Verification items for the finished model (mm, model axes). Face numbers are marked on the shaded views. A direction names the side the tool comes from. Round coordinates to 2 decimals unless told otherwise and drop trailing zeros. Order: outer loops, then holes, each group sorted by start corner. A loop starts at its lowest first (then second) coordinate and runs counter-clockwise, first axis right, second up. Notation, with made-up numbers: M 8.5,60 L 55.5,60 A36 ccw 55.5,99 Z; hole C 46.5,20.5 d7. An arc over 180 degrees is marked long. One line per item, written item: value. Start each with the question number.
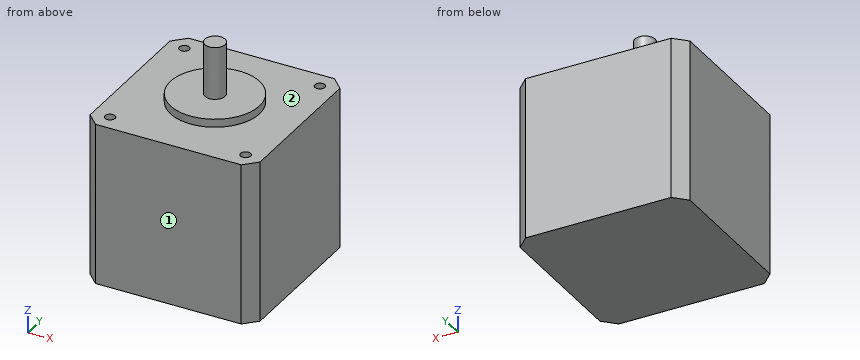
Autodesk Inventor part; units mm, degrees
ref_plane "YZ Plane" through (0, 0, 0) normal (1, 0, 0) x (0, 1, 0)
ref_plane "XZ Plane" through (0, 0, 0) normal (0, 1, 0) x (-1, 0, 0)
ref_plane "XY Plane" through (0, 0, 0) normal (0, 0, 1) x (1, 0, 0)
sketch "Sketch1" plane through (0, 0, 0) normal (0, 0, 1) x (1, 0, 0)
  line L0 (-3.9016, 5.1111) -> (32.0984, 5.1111)
  line L1 (35.0984, 2.1111) -> (35.0984, -33.8889)
  line L2 (32.0984, -36.8889) -> (-3.9016, -36.8889)
  line L3 (-6.9016, -33.8889) -> (-6.9016, 2.1111)
  circle A0 centre (14.0984, -15.8889) radius 11
  circle A1 centre (14.0984, -15.8889) radius 2.5
  line L4 (35.0984, 2.1111) -> (32.0984, 5.1111)
  line L5 (-6.9016, 2.1111) -> (-3.9016, 5.1111)
  line L6 (-6.9016, -33.8889) -> (-3.9016, -36.8889)
  line L7 (35.0984, -33.8889) -> (32.0984, -36.8889)
  circle A2 centre (30.8484, -32.6389) radius 1.25
  circle A3 centre (-2.6516, -32.6389) radius 1.25
  circle A4 centre (-2.6516, 0.8611) radius 1.25
  circle A5 centre (30.8484, 0.8611) radius 1.25
  point P0 (0, 0)
extrude "Extrusion1" add sketch "Sketch1" along normal blind 15 contours A1
extrude "Extrusion2" add sketch "Sketch1" along normal blind 2 contours A0
extrude "Extrusion3" add sketch "Sketch1" against normal blind 40 contours L0 L4 L1 L7 L2 L6 L3 L5 | A0 | A1 | A2 | A3 | A4 | A5
extrude "Extrusion4" cut sketch "Sketch1" against normal blind 5 contours A5
extrude "Extrusion5" cut sketch "Sketch1" against normal blind 5 contours A2
extrude "Extrusion6" cut sketch "Sketch1" against normal blind 5 contours A3
extrude "Extrusion7" cut sketch "Sketch1" against normal blind 5 contours A4
properties part number "motor" material "Iron, Malleable"
1. Tool access check on the marked faces 1 and 2. Record the directions out of +Z, -Z, +X, -X, +Y, -Y that give a thin tool (end or side, any length) a straight path to the whole face; none if there is none.
2. Scan lines: line 1 along Z through (x, y) = (-4, -30); line 2 along Z through (x, y) = (18, -26); line 3 along Y through (x, z) = (-4.5, -24.5). Record each from-to range of solid material in increasing order.
3. Section check D-D (z = 5.5). Record the cut outline in (x, y).
4. Depth check by flat-ended pin: pin 1 (3 mm diameter, centred on x = -3, y = 1.5, fed in from +Z); pin 2 (2 mm diameter, centred on x = 30.85, y = 0.86, fed in from +Z); pin 3 (6 mm diameter, centred on x = 25, z = 5.5, fed in from +Y). Enter the tip coordinate at first touch or a pass-through.
5. Section check A-A (y = -21). Record the cut outline in (x, z).
6. Section check C-C (y = -2). Record the cut outline in (x, z), and give its area (3 significant figures).
7. Section check B-B (x = 7). Record the cut outline in (y, z), and give its area (3 significant figures).
Geometry check:
1. face 1: +Z, -Z, +X, -X, -Y
1. face 2: +Z
2. line 1: z = -40 to 0
2. line 2: z = -40 to 2
2. line 3: y = -36.29 to 4.51
3. outline: C 14.1,-15.89 d5
4. pin 1: stops at z = 0
4. pin 2: stops at z = -5
4. pin 3: passes through
5. outline: M -6.9,-40 L 35.1,-40 L 35.1,0 L 23.84,0 L 23.84,2 L 4.36,2 L 4.36,0 L -6.9,0 Z
6. outline: M -6.9,-40 L 35.1,-40 L 35.1,0 L -6.9,0 Z
6. area: 1,680 mm²
7. outline: M -36.89,-40 L 5.11,-40 L 5.11,0 L -7.49,0 L -7.49,2 L -24.29,2 L -24.29,0 L -36.89,0 Z
7. area: 1,710 mm²
